Could you check a few things on this drawing? It's one solid part, dimensions in mm from its lowest x, y, z. A direction names the side the tool comes from. Give positions to 0.01 mm unless a question says otherwise; leave off trailing zeros. Loops run counter-clockwise (first coordinate to the right, second up) from the corner with the lowest first, then second, coordinate; pieces in that order, holes last. Notation, with made-up numbers: (6.25, -30) - (39.25, -30) arc R18 ccw to (39.25, 0) - close; hole circle Ø3 at (6, 9.25). An arc over 180 degrees is marked (long way). Use a Markdown table: item, result.
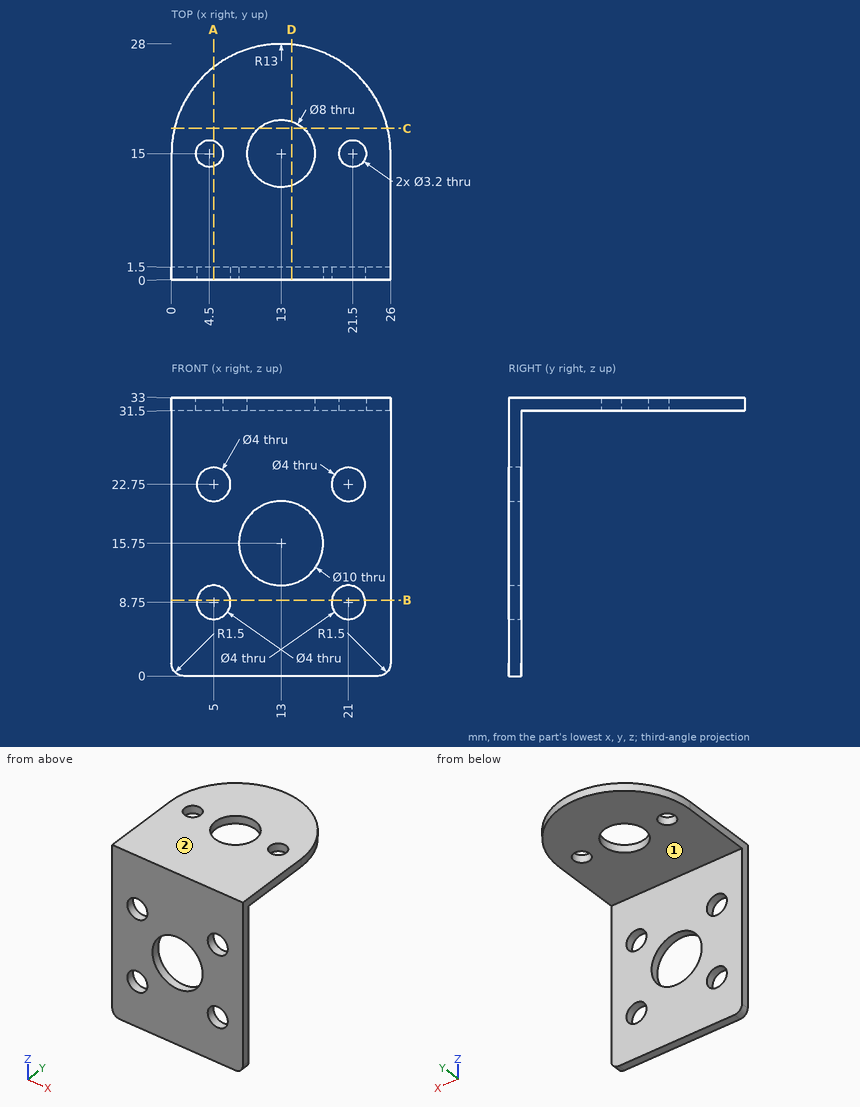
(1) Suppose I cut it at A-A on x = 5. Write out the boundary of the cut face in (y, z), plus the area to 3 significant figures.
A:
| item | result |
|---|---|
| outline | (0, 0) - (1.5, 0) - (1.5, 6.75) - (0, 6.75) - close; (0, 10.75) - (1.5, 10.75) - (1.5, 20.75) - (0, 20.75) - close; (0, 24.75) - (1.5, 24.75) - (1.5, 31.5) - (13.48, 31.5) - (13.48, 33) - (0, 33) - close; (16.52, 31.5) - (25.25, 31.5) - (25.25, 33) - (16.52, 33) - close |
| area | 68.6 mm2 |
(2) Suppose I cut it at C-C on y = 18. Write out the boundary of the cut face in (x, z).
A:
| item | result |
|---|---|
| outline | (0.35, 31.5) - (10.35, 31.5) - (10.35, 33) - (0.35, 33) - close; (15.65, 31.5) - (25.65, 31.5) - (25.65, 33) - (15.65, 33) - close |
(3) If I drill on line 1 (X direction, y = 0.5, z = 22.75); line 2 (Y direction, x = 16.25, z = 5); line 3 (Z direction, x = 11.75, y = 8), over which ranges is the centre line in solid material (lowest first)?
A:
| item | result |
|---|---|
| line 1 | 0 to 3, 7 to 19, 23 to 26 |
| line 2 | 0 to 1.5 |
| line 3 | 31.5 to 33 |
(4) Suppose I cut it at B-B on z = 9. Write out the boundary of the cut face in (x, y).
A:
| item | result |
|---|---|
| outline | (0, 0) - (3.02, 0) - (3.02, 1.5) - (0, 1.5) - close; (6.98, 0) - (19.02, 0) - (19.02, 1.5) - (6.98, 1.5) - close; (22.98, 0) - (26, 0) - (26, 1.5) - (22.98, 1.5) - close |
(5) On a 3-axis mill with a long thin cutter (end or side, diameter ignored), from which of +Z, -Z, +X, -X, +Y, -Y can I reach the whole of each face in a straight line? I mean the marked faces 1 and 2. Say none if no direction works.
A:
| item | result |
|---|---|
| face 1 | -Z, +X, -X, +Y |
| face 2 | +Z, +X, -X, +Y, -Y |
(6) Suppose I cut it at D-D on x = 14.25. Write out the boundary of the cut face in (y, z), plus the area to 3 significant figures.
A:
| item | result |
|---|---|
| outline | (0, 0) - (1.5, 0) - (1.5, 10.91) - (0, 10.91) - close; (0, 20.59) - (1.5, 20.59) - (1.5, 31.5) - (11.2, 31.5) - (11.2, 33) - (0, 33) - close; (18.8, 31.5) - (27.94, 31.5) - (27.94, 33) - (18.8, 33) - close |
| area | 63.2 mm2 |
(7) Will these pins go through, and if not, where does the flat tip stop? pin 1 (5 mm diameter, centred on x = 8, z = 9, fed in from +Y); pin 2 (3 mm diameter, centred on x = 11.5, y = 4.5, fed in from -Z).
A:
| item | result |
|---|---|
| pin 1 | y = 1.5 |
| pin 2 | z = 31.5 |
